from build123d import *

# Parameters (mm, degrees)
SKETCH1_R                                      = 38.1
BOSS_EXTRUDE1_DEPTH                            = 6.35
CBORE_FOR_4_BUTTON_HEAD_CAP_SCREW1_D           = 2.8702
CBORE_FOR_4_BUTTON_HEAD_CAP_SCREW1_CBORE_D     = 4.826
CBORE_FOR_4_BUTTON_HEAD_CAP_SCREW1_CBORE_DEPTH = 3.175
CIRPATTERN1_COUNT                              = 8


with BuildPart() as part:
    # Sketch1 → Boss-Extrude1 (new body)
    with BuildSketch(Plane(origin=(0, 0, 0), x_dir=(1, 0, 0), z_dir=(0, 1, 0))):
        Circle(SKETCH1_R)
    extrude(amount=BOSS_EXTRUDE1_DEPTH)

    # CBORE for #4 Button Head Cap Screw1 (through all)
    with Locations(Plane(origin=(0, 0, 0), x_dir=(-1, 0, 0), z_dir=(0, -1, 0))):
        with Locations((0, -33.3375)):
            cbore_for_4_button_head_cap_screw1 = CounterBoreHole(CBORE_FOR_4_BUTTON_HEAD_CAP_SCREW1_D / 2, CBORE_FOR_4_BUTTON_HEAD_CAP_SCREW1_CBORE_D / 2, CBORE_FOR_4_BUTTON_HEAD_CAP_SCREW1_CBORE_DEPTH)

    # CirPattern1: CBORE for #4 Button Head Cap Screw1 ×8 about axis
    cirpattern1_axis = Axis((0, 0, 0), (0, 1, 0))
    for i in range(1, CIRPATTERN1_COUNT):
        add(cbore_for_4_button_head_cap_screw1.rotate(cirpattern1_axis, i * 360 / CIRPATTERN1_COUNT), mode=Mode.SUBTRACT)


solid = part.part
Work out the finished part from the listing and answer in its coordinate system (mm). A direction names the side the tool comes from. Coordinates: 2 decimals unless noted, no trailing zeros. Write each loop counter-clockwise with the first axis right and the second up, starting at its lowest first coordinate (ties: lowest second). Pieces come first, ordered by that corner, then holes. Notation, with made-up numbers: M 71.25,54.25 L 85.25,54.25 A24 ccw 85.25,93.25 Z; hole C -2.5,-28 d4. An arc over 180 degrees is marked long. Write item = value, one per line.
1. Straight lines are drawn through the part: line 1 (Z direction, x = 0, y = 4.7); line 2 (X direction, y = 2, z = 0). For each, find the intervals that lie inside material, in ascending order. Write a range as from..to.
Solution:
line_1 = -38.1..-34.77, -31.9..31.9, 34.77..38.1
line_2 = -38.1..-35.75, -30.92..30.92, 35.75..38.1
2. For faces 1 (the face through (24.344, 4.785, 24.784)), 2 (the face through (1.297, 1.565, -31.303)), determine the directions among +Z, -Z, +X, -X, +Y, -Y from which every point of the face is accessible in a straight line to the end or side of a thin tool.
Solution:
face_1 = +Y, -Y
face_2 = -Y
3. Flat-ended cylindrical pins translate along their axes: pin 1 (4.5 mm diameter, centred on x = -23.57, z = -23.57, fed in from -Y) (3 decimals); pin 2 (1.5 mm diameter, centred on x = 26, y = 3, fed in from -Z); pin 3 (3 mm diameter, centred on x = 33.34, z = 0, fed in from +Y); pin 4 (1.5 mm diameter, centred on y = 4, z = -29.5, fed in from +X). Find the tip coordinate at first contact, or state that the pin passes through.
Solution:
pin_1 = 3.175
pin_2 = -28.53
pin_3 = 6.35
pin_4 = 25
4. Determine the mould class of faces 3 (the face through (-30.235, 3.131, 23.183)), 4 (the face through (-1, 6.35, -1)), 5 (the face through (31.303, 1.565, 1.297)) for opening direction Z: released by +Z, released by -Z, zero draft, split by the parting line, or undercut.
Solution:
face_3 = split by the parting line
face_4 = zero draft
face_5 = undercut
5. The part is cut by section C-C (z = -12). Determine the outline of the cut face in (x, y), then the cut area to 3 significant figures.
Solution:
outline = M -36.16,0 L 36.16,0 L 36.16,6.35 L -36.16,6.35 Z
area = 459 mm2
6. The part is cut by section D-D (x = -30). Determine the outline of the cut face in (y, z).
Solution:
outline = M 0,-23.49 L 6.35,-23.49 L 6.35,23.49 L 0,23.49 Z
7. The part is cut by section A-A (z = 0). State how many separate pieces and enclosed holes the cut face has, then the cut area to 3 significant figures.
Solution:
separate_pieces = 3
enclosed_holes = 0
area = 435 mm2
